from build123d import *

# Parameters (mm, degrees)
SKETCH_1_W          = 16.4
SKETCH_1_H          = 8.2
EXTRUDE_1_DEPTH     = 12.1
SKETCH_4_R          = 1.25
CUT_EXTRUDE_3_DEPTH = 8
CUT_EXTRUDE_4_DEPTH = 7.8
SKETCH_7_W          = 1
SKETCH_7_H          = 1
EXTRUDE_2_DEPTH     = 8
CHAMFER_1_SIZE      = 0.15
CHAMFER_2_SIZE      = 0.25
SKETCH_8_W          = 1
SKETCH_8_H          = 1
EXTRUDE_3_DEPTH     = 4
CHAMFER_3_SIZE      = 0.15
CHAMFER_4_SIZE      = 0.25
CHAMFER_6_SIZE      = 0.1
CHAMFER_7_SIZE      = 0.2
CHAMFER_8_SIZE      = 0.1
CHAMFER_9_SIZE      = 0.2


with BuildPart() as part:
    # Эскиз1 → Бобышка-Вытянуть1 (new body)
    with BuildSketch(Plane.XY):
        Rectangle(SKETCH_1_W, SKETCH_1_H)
    extrude(amount=EXTRUDE_1_DEPTH)

    # Эскиз4 → Вырез-Вытянуть3 (cut)
    with BuildSketch(Plane.XY.offset(12.1)):
        with Locations((-5, 0)):
            Circle(SKETCH_4_R)
        Circle(SKETCH_4_R)
        with Locations((5, 0)):
            Circle(SKETCH_4_R)
    extrude(amount=-CUT_EXTRUDE_3_DEPTH, mode=Mode.SUBTRACT)

    # Эскиз5 → Вырез-Вытянуть4 (cut)
    with BuildSketch(Plane.XY.offset(12.1)):
        with BuildLine():
            Line((-7.745621634, 0), (-7.745621634, 3.292901982))
            Line((-7.745621634, 3.292901982), (2.778509544, 3.292901982))
            Line((2.778509544, 3.292901982), (7.778509544, 3.292901982))
            Line((7.778509544, 3.292901982), (7.778509544, -2.548957219))
            Line((7.778509544, -2.548957219), (6.80582632, -2.548957219))
            ThreePointArc((6.80582632, -2.548957219), (5, -3.818893996), (3.19417368, -2.548957219))
            Line((3.19417368, -2.548957219), (1.80582632, -2.548957219))
            ThreePointArc((1.80582632, -2.548957219), (0, -3.818893996), (-1.80582632, -2.548957219))
            Line((-1.80582632, -2.548957219), (-3.19417368, -2.548957219))
            ThreePointArc((-3.19417368, -2.548957219), (-5, -3.818893996), (-6.80582632, -2.548957219))
            Line((-6.80582632, -2.548957219), (-7.745621634, -2.548957219))
            Line((-7.745621634, -2.548957219), (-7.745621634, 0))
        make_face()
    extrude(amount=-CUT_EXTRUDE_4_DEPTH, mode=Mode.SUBTRACT)

    # Эскиз7 → Бобышка-Вытянуть2 (add)
    with BuildSketch(Plane.XY.offset(4.1)):
        Rectangle(SKETCH_7_W, SKETCH_7_H)
        with Locations((-5, 0)):
            Rectangle(SKETCH_7_W, SKETCH_7_H)
        with Locations((5, 0)):
            Rectangle(SKETCH_7_W, SKETCH_7_H)
    extrude(amount=EXTRUDE_2_DEPTH)

    # Фаска1
    chamfer_1_edges = [part.edges().sort_by_distance(p)[0] for p in [
        (-4.5, -0.5, 8.1),
        (-4.5, 0.5, 8.1),
        (-5.5, 0.5, 8.1),
        (-5.5, -0.5, 8.1),
        (0.5, -0.5, 8.1),
        (0.5, 0.5, 8.1),
        (-0.5, 0.5, 8.1),
        (-0.5, -0.5, 8.1),
    ]]
    chamfer(chamfer_1_edges, length=CHAMFER_1_SIZE)

    # Фаска2
    # the kernel refuses this chamfer: 0.25 mm, written as the material it takes off along each edge
    with BuildSketch(Plane(origin=(-0.5, -0.992920747, 12.1), x_dir=(-0.027495876610586414, 0, -0.9996219169112968), z_dir=(0, 1, 0)), Plane(origin=(-0.992920747, 0.5, 12.1), x_dir=(0, 0.027495876610586414, -0.9996219169112968), z_dir=(1, 0, 0)), Plane(origin=(0.5, 0.992920747, 12.1), x_dir=(0.027495876610586414, 0, -0.9996219169112968), z_dir=(0, -1, 0)), Plane(origin=(0.992920747, -0.5, 12.1), x_dir=(0, -0.027495876610586414, -0.9996219169112968), z_dir=(-1, 0, 0)), Plane(origin=(-4.5, 0.992920747, 12.1), x_dir=(0.02749587661058555, 0, -0.9996219169112968), z_dir=(0, -1, 0)), Plane(origin=(-4.007079253, -0.5, 12.1), x_dir=(0, -0.027495876610586414, -0.9996219169112968), z_dir=(-1, 0, 0)), Plane(origin=(-5.5, -0.992920747, 12.1), x_dir=(-0.02749587661058555, 0, -0.9996219169112968), z_dir=(0, 1, 0)), Plane(origin=(-5.992920747, 0.5, 12.1), x_dir=(0, 0.027495876610586414, -0.9996219169112968), z_dir=(1, 0, 0))) as chamfer_2_piece_1:
        Polygon((CHAMFER_2_SIZE * 0.999621916911, -CHAMFER_2_SIZE * 0.0274958766106), (-CHAMFER_2_SIZE * 0.0274958766106, -CHAMFER_2_SIZE * 0.999621916911), (0, 0), align=None)
    extrude(amount=1.985841494, mode=Mode.SUBTRACT)

    # Эскиз8 → Бобышка-Вытянуть3 (add)
    with BuildSketch(Plane(origin=(0, -4.1, 0), x_dir=(-1, 0, 0), z_dir=(0, -1, 0))):
        with Locations((0, -1.6)):
            Rectangle(SKETCH_8_W, SKETCH_8_H)
        with Locations((5, -1.6)):
            Rectangle(SKETCH_8_W, SKETCH_8_H)
        with Locations((-5, -1.6)):
            Rectangle(SKETCH_8_W, SKETCH_8_H)
    extrude(amount=EXTRUDE_3_DEPTH)

    # Фаска3
    chamfer_3_edges = [part.edges().sort_by_distance(p)[0] for p in [
        (-4.5, -6.1, 1.1),
        (-4.5, -6.1, 2.1),
        (-5.5, -6.1, 2.1),
        (-5.5, -6.1, 1.1),
        (0.5, -6.1, 1.1),
        (0.5, -6.1, 2.1),
        (-0.5, -6.1, 2.1),
        (-0.5, -6.1, 1.1),
    ]]
    chamfer(chamfer_3_edges, length=CHAMFER_3_SIZE)

    # Фаска4
    # the kernel refuses this chamfer: 0.25 mm, written as the material it takes off along each edge
    with BuildSketch(Plane(origin=(0.5, -8.1, 2.592920747), x_dir=(0.02749587661058651, 0.9996219169112968, 0), z_dir=(0, 0, -1)), Plane(origin=(-0.5, -8.1, 0.607079253), x_dir=(-0.02749587661058651, 0.9996219169112968, 0), z_dir=(0, 0, 1)), Plane(origin=(-0.992920747, -8.1, 2.1), x_dir=(0, 0.9996219169112968, 0.027495876610585647), z_dir=(1, 0, 0)), Plane(origin=(0.992920747, -8.1, 1.1), x_dir=(0, 0.9996219169112968, -0.02749587661058651), z_dir=(-1, 0, 0)), Plane(origin=(-5.5, -8.1, 0.607079253), x_dir=(-0.027495876610585647, 0.9996219169112968, 0), z_dir=(0, 0, 1)), Plane(origin=(-5.992920747, -8.1, 2.1), x_dir=(0, 0.9996219169112968, 0.027495876610585647), z_dir=(1, 0, 0)), Plane(origin=(-4.5, -8.1, 2.592920747), x_dir=(0.027495876610585647, 0.9996219169112968, 0), z_dir=(0, 0, -1)), Plane(origin=(-4.007079253, -8.1, 1.1), x_dir=(0, 0.9996219169112968, -0.02749587661058651), z_dir=(-1, 0, 0))) as chamfer_4_piece_1:
        Polygon((CHAMFER_4_SIZE * 0.999621916911, -CHAMFER_4_SIZE * 0.0274958766106), (-CHAMFER_4_SIZE * 0.0274958766106, -CHAMFER_4_SIZE * 0.999621916911), (0, 0), align=None)
    extrude(amount=1.985841494, mode=Mode.SUBTRACT)

    # Фаска6
    chamfer_6_edges = [part.edges().sort_by_distance(p)[0] for p in [
        (5.5, -0.5, 8.1),
        (5.5, 0.5, 8.1),
        (4.5, 0.5, 8.1),
        (4.5, -0.5, 8.1),
    ]]
    chamfer(chamfer_6_edges, length=CHAMFER_6_SIZE)

    # Фаска7
    # the kernel refuses this chamfer: 0.2 mm, written as the material it takes off along each edge
    with BuildSketch(Plane(origin=(5.5, 0.914336598, 12.1), x_dir=(0.02749587661058742, 0, -0.9996219169112966), z_dir=(0, -1, 0)), Plane(origin=(5.914336598, -0.5, 12.1), x_dir=(0, -0.02749587661058634, -0.9996219169112966), z_dir=(-1, 0, 0)), Plane(origin=(4.5, -0.914336598, 12.1), x_dir=(-0.02749587661058742, 0, -0.9996219169112966), z_dir=(0, 1, 0)), Plane(origin=(4.085663402, 0.5, 12.1), x_dir=(0, 0.02749587661058634, -0.9996219169112966), z_dir=(1, 0, 0))) as chamfer_7_piece_1:
        Polygon((CHAMFER_7_SIZE * 0.999621916911, -CHAMFER_7_SIZE * 0.0274958766106), (-CHAMFER_7_SIZE * 0.0274958766106, -CHAMFER_7_SIZE * 0.999621916911), (0, 0), align=None)
    extrude(amount=1.828673195, mode=Mode.SUBTRACT)

    # Фаска8
    chamfer_8_edges = [part.edges().sort_by_distance(p)[0] for p in [
        (5.5, -6.1, 1.1),
        (5.5, -6.1, 2.1),
        (4.5, -6.1, 2.1),
        (4.5, -6.1, 1.1),
    ]]
    chamfer(chamfer_8_edges, length=CHAMFER_8_SIZE)

    # Фаска9
    # the kernel refuses this chamfer: 0.2 mm, written as the material it takes off along each edge
    with BuildSketch(Plane(origin=(5.5, -8.1, 2.514336598), x_dir=(0.027495876610587302, 0.9996219169112966, 0), z_dir=(0, 0, -1)), Plane(origin=(5.914336598, -8.1, 1.1), x_dir=(0, 0.9996219169112968, -0.027495876610586226), z_dir=(-1, 0, 0)), Plane(origin=(4.5, -8.1, 0.685663402), x_dir=(-0.027495876610587302, 0.9996219169112966, 0), z_dir=(0, 0, 1)), Plane(origin=(4.085663402, -8.1, 2.1), x_dir=(0, 0.9996219169112966, 0.027495876610587302), z_dir=(1, 0, 0))) as chamfer_9_piece_1:
        Polygon((CHAMFER_9_SIZE * 0.999621916911, -CHAMFER_9_SIZE * 0.0274958766106), (-CHAMFER_9_SIZE * 0.0274958766106, -CHAMFER_9_SIZE * 0.999621916911), (0, 0), align=None)
    extrude(amount=1.828673195, mode=Mode.SUBTRACT)


solid = part.part
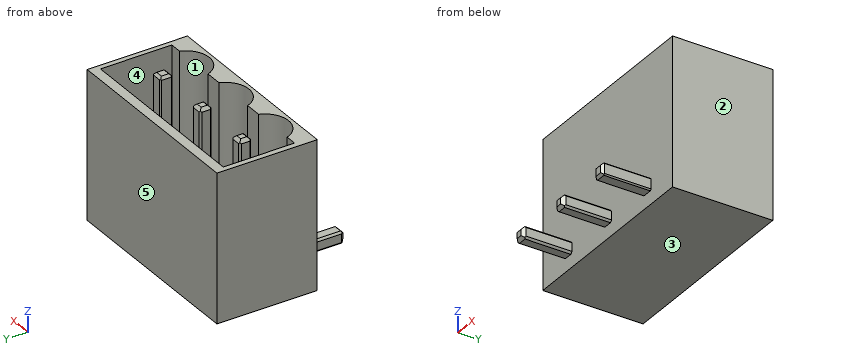
The model under review builds one solid part; all positions refer to its coordinate system, in mm. Face numbers are marked on the shaded views. A direction names the side the tool comes from. Round coordinates to 2 decimals unless told otherwise and drop trailing zeros. Order: outer loops, then holes, each group sorted by start corner. A loop starts at its lowest first (then second) coordinate and runs counter-clockwise, first axis right, second up. Notation, with made-up numbers: (65, 82) -> (74, 82) arc R27 cw to (74, 103) -> close; hole circle Ø3 at (-35.75, -6). An arc over 180 degrees is marked (long way). Write item = value, one per line. Start each with the question number.
Item 1: Mouldability with a two-part tool opening along X and no side actions: class the marked faces 1, 2 and 3 as released by +X, released by -X, zero draft, split by the parting line, or undercut.
Item 2: For line 1 along Y through (x, z) = (-5, 4.15); line 2 along X through (y, z) = (0, 9); line 3 along X through (y, z) = (1, 11), list the stretches that pass through material, from the lowest coordinate up.
Item 3: Clearance check with flat-ended pins moving along their axes: pin 1 Ø0.6 at (y, z) = (-6.5, 1.5) entering from -X; pin 2 Ø0.8 at (x, y) = (-5, -6.5) entering from +Z; pin 3 Ø3 at (x, z) = (3.5, 7) entering from -Y; pin 4 Ø1.5 at (x, y) = (-3.5, -5) entering from +Z. State where each tip first meets the part, or that it passes through.
Item 4: Consider section D-D on z = 3. Write out the cut boundary in (x, y), plus the area to 3 significant figures.
Item 5: For the marked faces 4 and 5, list the 3-axis set-ups (+Z, -Z, +X, -X, +Y, -Y) from which the entire face can be reached by the end or side of a thin tool; tool diameter is ignored.
Item 6: Consider section B-B on x = 0. Write out the cut boundary in (y, z), plus the area to 3 significant figures.
Item 7: Consider section C-C on z = 8.25. Count the separate pieces of the cut face and the enclosed holes in it, plus the area to 3 significant figures.
Item 8: Consider section A-A on y = -5.25. Write out the cut boundary in (x, z).
Conclusion:
q1.face_1 = undercut
q1.face_2 = released by +X
q1.face_3 = zero draft
q2.line_1 = -4.1 to -1.25, -0.5 to 0.5, 1.25 to 4.1
q2.line_2 = -8.2 to -7.75, -5.5 to -4.5, -0.5 to 0.5, 4.5 to 5.5, 7.78 to 8.2
q2.line_3 = -8.2 to -7.75, 7.78 to 8.2
q3.pin_1 = -5.5
q3.pin_2 = 2.1
q3.pin_3 = -4.1
q3.pin_4 = through
q4.outline = (-8.2, -4.1) -> (8.2, -4.1) -> (8.2, 4.1) -> (-8.2, 4.1) -> close
q4.area = 134 mm2
q5.face_4 = +Z
q5.face_5 = +Z, -Z, +X, -X, +Y
q6.outline = (-8.1, 1.35) -> (-7.85, 1.1) -> (-4.1, 1.1) -> (-4.1, 0) -> (4.1, 0) -> (4.1, 12.1) -> (3.29, 12.1) -> (3.29, 4.3) -> (1.25, 4.3) -> (1.25, 4.1) -> (0.5, 4.1) -> (0.5, 11.85) -> (0.25, 12.1) -> (-0.25, 12.1) -> (-0.5, 11.85) -> (-0.5, 4.1) -> (-1.25, 4.1) -> (-1.25, 4.3) -> (-3.82, 4.3) -> (-3.82, 12.1) -> (-4.1, 12.1) -> (-4.1, 2.1) -> (-7.85, 2.1) -> (-8.1, 1.85) -> close
q6.area = 55.1 mm2
q7.separate_pieces = 4
q7.enclosed_holes = 1
q7.area = 36.7 mm2
q8.outline = (-5.5, 1.25) -> (-5.35, 1.1) -> (-4.65, 1.1) -> (-4.5, 1.25) -> (-4.5, 1.95) -> (-4.65, 2.1) -> (-5.35, 2.1) -> (-5.5, 1.95) -> close; (-0.5, 1.25) -> (-0.35, 1.1) -> (0.35, 1.1) -> (0.5, 1.25) -> (0.5, 1.95) -> (0.35, 2.1) -> (-0.35, 2.1) -> (-0.5, 1.95) -> close; (4.5, 1.2) -> (4.6, 1.1) -> (5.4, 1.1) -> (5.5, 1.2) -> (5.5, 2) -> (5.4, 2.1) -> (4.6, 2.1) -> (4.5, 2) -> close
